```python
from build123d import *

# Parameters (mm, degrees)
SKETCH1_R               = 3
BOSS_EXTRUDE1_DEPTH     = 11.938
CUT_EXTRUDE1_DEPTH      = 58.922498599
CUT_EXTRUDE1_DEPTH_BACK = 10.3378
FILLET1_R               = 3.175


with BuildPart() as part:
    # Sketch1 → Boss-Extrude1 (new body)
    with BuildSketch(Plane(origin=(0, 0, 0), x_dir=(1, 0, 0), z_dir=(0, 1, 0))):
        with BuildLine():
            Line((-31.5, -42.5), (31.5, -42.5))
            ThreePointArc((31.5, -42.5), (35.742640687, -40.742640687), (37.5, -36.5))
            Line((37.5, -36.5), (37.5, 36.5))
            ThreePointArc((37.5, 36.5), (35.742640687, 40.742640687), (31.5, 42.5))
            Line((31.5, 42.5), (-31.5, 42.5))
            ThreePointArc((-31.5, 42.5), (-35.742640687, 40.742640687), (-37.5, 36.5))
            Line((-37.5, 36.5), (-37.5, -36.5))
            ThreePointArc((-37.5, -36.5), (-35.742640687, -40.742640687), (-31.5, -42.5))
        make_face()
        with Locations(Location((-31.5, 36.5, 0), (0, 0, 270))):
            Circle(SKETCH1_R, mode=Mode.SUBTRACT)
        with Locations(Location((-31.5, -36.5, 0), (0, 0, 270))):
            Circle(SKETCH1_R, mode=Mode.SUBTRACT)
        with Locations(Location((31.5, -36.5, 0), (0, 0, 270))):
            Circle(SKETCH1_R, mode=Mode.SUBTRACT)
        with Locations(Location((31.5, 36.5, 0), (0, 0, 270))):
            Circle(SKETCH1_R, mode=Mode.SUBTRACT)
    extrude(amount=-BOSS_EXTRUDE1_DEPTH)

    # Sketch2 → Cut-Extrude1 (cut, two sides: drawn at the far end of the back side and taken through both)
    with BuildSketch(Plane(origin=(0, 0, 0), x_dir=(1, 0, 0), z_dir=(0, 1, 0)).offset(-CUT_EXTRUDE1_DEPTH_BACK)):
        with BuildLine():
            Line((-22.891864313, -36.5), (22.891864313, -36.5))
            ThreePointArc((22.891864313, -36.5), (24.707385496, -35.929708781), (25.870701458, -34.423705722))
            ThreePointArc((25.870701458, -34.423705722), (27.257359313, -32.257359313), (29.423705722, -30.870701458))
            ThreePointArc((29.423705722, -30.870701458), (30.929708781, -29.707385496), (31.5, -27.891864313))
            Line((31.5, -27.891864313), (31.5, 27.891864313))
            ThreePointArc((31.5, 27.891864313), (30.929708781, 29.707385496), (29.423705722, 30.870701458))
            ThreePointArc((29.423705722, 30.870701458), (27.257359313, 32.257359313), (25.870701458, 34.423705722))
            ThreePointArc((25.870701458, 34.423705722), (24.707385496, 35.929708781), (22.891864313, 36.5))
            Line((22.891864313, 36.5), (-22.891864313, 36.5))
            ThreePointArc((-22.891864313, 36.5), (-24.707385496, 35.929708781), (-25.870701458, 34.423705722))
            ThreePointArc((-25.870701458, 34.423705722), (-27.257359313, 32.257359313), (-29.423705722, 30.870701458))
            ThreePointArc((-29.423705722, 30.870701458), (-30.929708781, 29.707385496), (-31.5, 27.891864313))
            Line((-31.5, 27.891864313), (-31.5, -27.891864313))
            ThreePointArc((-31.5, -27.891864313), (-30.929708781, -29.707385496), (-29.423705722, -30.870701458))
            ThreePointArc((-29.423705722, -30.870701458), (-27.257359313, -32.257359313), (-25.870701458, -34.423705722))
            ThreePointArc((-25.870701458, -34.423705722), (-24.707385496, -35.929708781), (-22.891864313, -36.5))
        make_face()
    extrude(amount=CUT_EXTRUDE1_DEPTH + CUT_EXTRUDE1_DEPTH_BACK, mode=Mode.SUBTRACT)

    # Fillet1
    fillet1_edges = [part.edges().sort_by_distance(p)[0] for p in [
        (24.707385496, -10.3378, -35.929708781),
        (27.257359313, -10.3378, -32.257359313),
        (30.929708781, -10.3378, -29.707385496),
        (31.5, -10.3378, 0),
        (30.929708781, -10.3378, 29.707385496),
        (27.257359313, -10.3378, 32.257359313),
        (24.707385496, -10.3378, 35.929708781),
        (0, -10.3378, 36.5),
        (-24.707385496, -10.3378, 35.929708781),
        (-27.257359313, -10.3378, 32.257359313),
        (-30.929708781, -10.3378, 29.707385496),
        (-31.5, -10.3378, 0),
        (-30.929708781, -10.3378, -29.707385496),
        (-27.257359313, -10.3378, -32.257359313),
        (-24.707385496, -10.3378, -35.929708781),
        (0, -10.3378, -36.5),
    ]]
    fillet(fillet1_edges, radius=FILLET1_R)


solid = part.part
```
Here's how the part is built. I have some questions about the finished solid (model axes, mm). A direction names the side the tool comes from. Give positions to 0.01 mm unless a question says otherwise; leave off trailing zeros. Write each loop counter-clockwise with the first axis right and the second up, starting at its lowest first coordinate (ties: lowest second). Pieces come first, ordered by that corner, then holes. Notation, with made-up numbers: M -2.75,34.5 L 22.25,34.5 A16 ccw 22.25,59.5 Z; hole C 38,-32.75 d10. An arc over 180 degrees is marked long. Put each result on its own line as item: value. Start each with the question number.
Item 1: I need wall thicknesses on L1, parallel to X at y = -8.5, z = -36.5; L2, parallel to X at y = -3.75, z = 15; L3, parallel to Z at x = 10.5, y = -6.5. Which ranges of each line are inside material? Lowest first, please. Write a range as from..to.
Item 2: If we section it at A-A, the plane y = -5.5: Write out the boundary of the cut face in (x, z) (3 decimals).
Item 3: If we section it at C-C, the plane x = -30.5: Write out the boundary of the cut face in (y, z), then the cut area to 3 significant figures.
Item 4: If we section it at D-D, the plane x = -20: Write out the boundary of the cut face in (y, z) (3 decimals), then the cut area to 3 significant figures.
Item 5: Thinking about a two-plate mould opening in Z: for faces 1 (the flat face through (0, -6, 42.5)), 2 (the cylindrical face through (27.232, -3.632, 32.283)), 3 (the flat face through (0, -6, -42.5)), 4 (the flat face through (-31.5, -4, 0)), which applies, +Z half, -Z half, draft (parallel to the pull), parting line (faces both ways), or undercut?
Item 6: If we section it at B-B, the plane z = 37.5: Write out the boundary of the cut face in (x, y), then the cut area to 3 significant figures.
Item 7: Will these pins go through, and if not, where does the flat tip stop? pin 1 (3 mm diameter, centred on x = -20.5, z = -34, fed in from +Y); pin 2 (3 mm diameter, centred on x = 19.5, z = 19, fed in from +Y).
Item 8: On a 3-axis mill with a long thin cutter (end or side, diameter ignored), from which of +Z, -Z, +X, -X, +Y, -Y can I reach the whole of each face in a straight line? I mean faces 5 (the flat face through (-1, -11.938, -1)), 6 (the cylindrical face through (24.685, -3.632, 35.945)). Say none if no direction works.
Values:
1. L1: -37.5..-34.5, -28.5..28.5, 34.5..37.5
1. L2: -37.5..-31.5, 31.5..37.5
1. L3: -42.5..-36.5, 36.5..42.5
2. outline: M -37.5,-36.5 A6 ccw -31.5,-42.5 L 31.5,-42.5 A6 ccw 37.5,-36.5 L 37.5,36.5 A6 ccw 31.5,42.5 L -31.5,42.5 A6 ccw -37.5,36.5 Z; hole C -31.5,-36.5 d6; hole C -31.5,36.5 d6; hole M -31.5,-27.892 A3.175 ccw -29.424,-30.871 A6 cw -25.871,-34.424 A3.175 ccw -22.892,-36.5 L 22.892,-36.5 A3.175 ccw 25.871,-34.424 A6 cw 29.424,-30.871 A3.175 ccw 31.5,-27.892 L 31.5,27.892 A3.175 ccw 29.424,30.871 A6 cw 25.871,34.424 A3.175 ccw 22.892,36.5 L -22.892,36.5 A3.175 ccw -25.871,34.424 A6 cw -29.424,30.871 A3.175 ccw -31.5,27.892 Z; hole C 31.5,-36.5 d6; hole C 31.5,36.5 d6
3. outline: M -11.94,-42.5 L 0,-42.5 L 0,-39.33 L -11.94,-39.33 Z; M -11.94,-33.67 L 0,-33.67 L 0,-30.2 L -7.16,-30.2 A2.31 cw -9.48,-27.89 L -9.48,27.89 A2.31 cw -7.16,30.2 L 0,30.2 L 0,33.67 L -11.94,33.67 Z; M -11.94,39.33 L 0,39.33 L 0,42.5 L -11.94,42.5 Z
3. area: 310 mm²
4. outline: M -11.938,-42.5 L 0,-42.5 L 0,-36.5 L -7.163,-36.5 A3.175 cw -10.338,-33.325 L -10.338,33.325 A3.175 cw -7.163,36.5 L 0,36.5 L 0,42.5 L -11.938,42.5 Z
4. area: 264 mm²
5. face 1: +Z half
5. face 2: undercut
5. face 3: -Z half
5. face 4: undercut
6. outline: M -37.42,-11.94 L -34.33,-11.94 L -34.33,0 L -37.42,0 Z; M -28.67,-11.94 L 28.67,-11.94 L 28.67,0 L -28.67,0 Z; M 34.33,-11.94 L 37.42,-11.94 L 37.42,0 L 34.33,0 Z
6. area: 758 mm²
7. pin 1: y = -9.48
7. pin 2: y = -10.34
8. face 5: +Z, -Z, +X, -X, -Y
8. face 6: +Y
